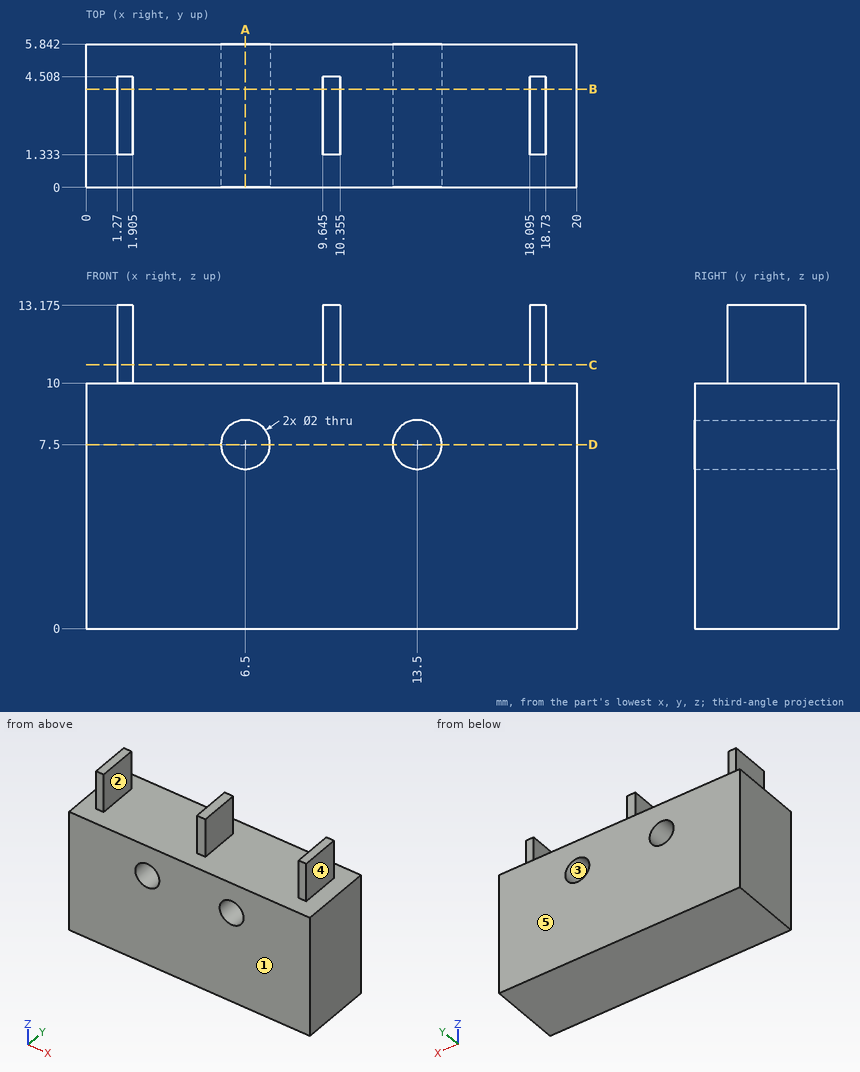
Check sheet for the drawn part. Datum: minimum x, y, z corner. Units: mm. A direction names the side the tool comes from. Round coordinates to 2 decimals unless told otherwise and drop trailing zeros. Write each loop counter-clockwise with the first axis right and the second up, starting at its lowest first coordinate (ties: lowest second). Pieces come first, ordered by that corner, then holes. Notation, with made-up numbers: (38.5, 72) -> (90.5, 72) arc R16 cw to (90.5, 85) -> close; hole circle Ø7 at (-30, 16). An arc over 180 degrees is marked (long way). One line per item, written item: value. Start each with the question number.
(1) Scan lines: line 1 (X direction, y = 4.6, z = 7.5); line 2 (Z direction, x = 6.5, y = 3.9); line 3 (Z direction, x = 3, y = 1.7). Record each from-to range of solid material in increasing order. Write a range as [from, to].
(2) Cross-section at B-B, the plane y = 4. Record the cut outline in (x, z) (1 decimal), and give its area (3 significant figures).
(3) Cross-section at D-D, the plane z = 7.5. Record the cut outline in (x, y).
(4) Cross-section at C-C, the plane z = 10.75. Record the cut outline in (x, y) (1 decimal).
(5) Draft check along X on the marked faces 3, 4 and 5. Enter one of: +X half, -X half, draft (parallel to the pull), parting line (faces both ways), or undercut.
(6) Go/stop test with flat-tipped pins: pin 1 Ø2 at (x, y) = (8.5, 4.5) entering from +Z; pin 2 Ø1 at (y, z) = (3, 11.5) entering from -X; pin 3 Ø1.8 at (x, z) = (6.5, 7.5) entering from +Y; pin 4 Ø1 at (y, z) = (3.5, 12.5) entering from +X. Record where each tip stops, or that it passes through.
(7) Access from +Z, -Z, +X, -X, +Y, -Y to the whole of each face (thin tool, end or side, straight path). Record for the marked faces 1 and 2.
(8) Cross-section at A-A, the plane x = 6.5. Record the cut outline in (y, z).
Answer:
1. line 1: [0, 5.5], [7.5, 12.5], [14.5, 20]
1. line 2: [0, 6.5], [8.5, 10]
1. line 3: [0, 10]
2. outline: (0, 0) -> (20, 0) -> (20, 10) -> (18.7, 10) -> (18.7, 13.2) -> (18.1, 13.2) -> (18.1, 10) -> (10.4, 10) -> (10.4, 13.2) -> (9.6, 13.2) -> (9.6, 10) -> (1.9, 10) -> (1.9, 13.2) -> (1.3, 13.2) -> (1.3, 10) -> (0, 10) -> close; hole circle Ø2 at (6.5, 7.5); hole circle Ø2 at (13.5, 7.5)
2. area: 200 mm²
3. outline: (0, 0) -> (5.5, 0) -> (5.5, 5.84) -> (0, 5.84) -> close; (7.5, 0) -> (12.5, 0) -> (12.5, 5.84) -> (7.5, 5.84) -> close; (14.5, 0) -> (20, 0) -> (20, 5.84) -> (14.5, 5.84) -> close
4. outline: (1.3, 1.3) -> (1.9, 1.3) -> (1.9, 4.5) -> (1.3, 4.5) -> close; (9.6, 1.3) -> (10.4, 1.3) -> (10.4, 4.5) -> (9.6, 4.5) -> close; (18.1, 1.3) -> (18.7, 1.3) -> (18.7, 4.5) -> (18.1, 4.5) -> close
5. face 3: undercut
5. face 4: +X half
5. face 5: draft
6. pin 1: z = 10
6. pin 2: x = 1.27
6. pin 3: through
6. pin 4: x = 18.73
7. face 1: +Z, -Z, +X, -X, -Y
7. face 2: +Z, +Y, -Y
8. outline: (0, 0) -> (5.84, 0) -> (5.84, 6.5) -> (0, 6.5) -> close; (0, 8.5) -> (5.84, 8.5) -> (5.84, 10) -> (0, 10) -> close
